from build123d import *

# Parameters (mm, degrees)
F0_W     = 2
F0_H     = 7.224001
F1_DEPTH = 50
F2_W     = 40
F2_H     = 10.308505
F3_DEPTH = 12.5


with BuildPart() as f1:
    # F0 (on Right) → F1 (new body)
    with BuildSketch(Plane.YZ):
        Polygon((-4.891242, 2), (-4.891242, 0), (3.108758, 0), (3.108758, 2), (1.108758, 2), (-1.891242, 2), (-3.891242, 2), align=None)
        with Locations((-2.891242, 5.612)):
            Rectangle(F0_W, F0_H)
        with Locations((2.108758, 5.612)):
            Rectangle(F0_W, F0_H)
    extrude(amount=F1_DEPTH)

    # F2 (on Front) → F3 (cut, symmetric)
    with BuildSketch(Plane.XZ):
        with Locations((25, 7.154253)):
            Rectangle(F2_W, F2_H)
    extrude(amount=F3_DEPTH, both=True, mode=Mode.SUBTRACT)


with BuildPart() as f1_1:
    # F4: moved
    add(f1.part.moved(Location((-25, 0, 0))))


solid = f1_1.part
Design review of the part built by this model. Coordinates are the model's own, in mm. A direction names the side the tool comes from. Coordinates: 2 decimals unless noted, no trailing zeros. Loops run counter-clockwise (first coordinate to the right, second up) from the corner with the lowest first, then second, coordinate; pieces in that order, holes last. Notation, with made-up numbers: (51, 6.5) -> (109, 6.5) arc R8 cw to (109, 16.5) -> close; hole circle Ø7 at (79, 2.25). An arc over 180 degrees is marked (long way). Use a Markdown table: item, result. Add a question column.
Item 1: Clearance check with a flat-ended pin moving along its axis: P1, Ø3.5, axis at x = -9.5, y = 0, coming from the +Z side. State where the tip first meets the part, or that it passes through.
Item 2: We need section A-A, the plane z = 5.5. Write out the cut boundary in (x, y).
Item 3: Wall thickness on L1, parallel to X at y = -2.25, z = 8; L2, parallel to Z at x = 1.5, y = -0.75; L3, parallel to Y at x = 20.5, z = 2.75: over which ranges is each line inside the solid? List them lowest first. Write a range as from..to.
Item 4: We need section C-C, the plane y = -3.25. Write out the cut boundary in (x, z).
Item 5: We need section B-B, the plane x = 21.5. Write out the cut boundary in (y, z), and give its area (3 significant figures).
Item 6: Machinability: for faces 4 (the flat face through (20, -3, 6)), 5 (the flat face through (-0.4, -4.4, 2)), 6 (the flat face through (-25, -3, 4)), 7 (the flat face through (25, -3, 4)), 8 (the flat face through (0, 0, 2)), which of the approach directions +Z, -Z, +X, -X, +Y, -Y give a long, thin tool a straight path to every point of the face, cutting with its end or side? Answer none if there is none.
Item 7: We need section D-D, the plane y = -0.5. Write out the cut boundary in (x, z).
Item 8: The part is to be moulded in two halves that separate along Y. For faces 1 (the flat face through (-23, -3, 9.224)), 2 (the flat face through (-20.5, -1.891, 5.6)), 3 (the flat face through (0, 3.109, 1)), say which applies: +Y half, -Y half, draft (parallel to the pull), parting line (faces both ways), or undercut.
Numbers:
| question | item | result |
|---|---|---|
| 1 | P1 | stops at z = 2 |
| 2 | outline | (-25, -3.89) -> (-20, -3.89) -> (-20, -1.89) -> (-25, -1.89) -> close; (-25, 1.11) -> (-20, 1.11) -> (-20, 3.11) -> (-25, 3.11) -> close; (20, -3.89) -> (25, -3.89) -> (25, -1.89) -> (20, -1.89) -> close; (20, 1.11) -> (25, 1.11) -> (25, 3.11) -> (20, 3.11) -> close |
| 3 | L1 | x = -25..-20, 20..25 |
| 3 | L2 | z = 0..2 |
| 3 | L3 | y = -3.89..-1.89, 1.11..3.11 |
| 4 | outline | (-25, 0) -> (25, 0) -> (25, 9.22) -> (20, 9.22) -> (20, 2) -> (-20, 2) -> (-20, 9.22) -> (-25, 9.22) -> close |
| 5 | outline | (-4.89, 0) -> (3.11, 0) -> (3.11, 9.22) -> (1.11, 9.22) -> (1.11, 2) -> (-1.89, 2) -> (-1.89, 9.22) -> (-3.89, 9.22) -> (-3.89, 2) -> (-4.89, 2) -> close |
| 5 | area | 44.9 mm^2 |
| 6 | face 4 | +Z, +Y, -Y |
| 6 | face 5 | +Z, +X, -X, -Y |
| 6 | face 6 | +Z, -Z, -X, +Y, -Y |
| 6 | face 7 | +Z, -Z, +X, +Y, -Y |
| 6 | face 8 | +Z, +X, -X |
| 7 | outline | (-25, 0) -> (25, 0) -> (25, 2) -> (-25, 2) -> close |
| 8 | face 1 | draft |
| 8 | face 2 | undercut |
| 8 | face 3 | +Y half |
